Input: part model. Units: mm. Frame: model coordinates. A direction names the side the tool comes from. Coordinates: 2 decimals unless noted, no trailing zeros. Order: outer loops, then holes, each group sorted by start corner. A loop starts at its lowest first (then second) coordinate and runs counter-clockwise, first axis right, second up. Notation, with made-up numbers: M 60,23 L 87,23 A33 ccw 87,56 Z; hole C -39.75,18 d5. An arc over 180 degrees is marked long. One line per item, written item: value.
```python
from build123d import *

# Parameters (mm, degrees)
F0_W        = 16
F0_H        = 22
F0_W_2      = 4
F0_H_2      = 9
F1_DEPTH    = 3
F2_DEPTH    = 15
F3_DEPTH    = 2.5
F4_DEPTH    = 2.5
F5_T1_DEPTH = 3
F5_T3_DEPTH = 25
F7_W        = 4
F7_H        = 9
F8_DEPTH    = 1
F10_DEPTH   = 1
F11_R       = 5


# Not quite as in the source:
# - a fillet or chamfer that OpenCascade refuses, or shapes differently, is made with other operations: its cross-section is extruded or revolved along the edge and cut away or added
# - two fillets or chamfers of one size are made in one step


with BuildPart() as f1:
    # F0 (on Top) → F1 (new body)
    with BuildSketch(Plane.XY):
        with Locations((8, 11)):
            Rectangle(F0_W, F0_H)
        with Locations((6, 9.5)):
            Rectangle(F0_W_2, F0_H_2, mode=Mode.SUBTRACT)
        with Locations((24, 11)):
            Rectangle(F0_W, F0_H)
        with Locations((26, 9.5)):
            Rectangle(F0_W_2, F0_H_2, mode=Mode.SUBTRACT)
    extrude(amount=F1_DEPTH)

    # F0 (on Top) → F2 (join)
    with BuildSketch(Plane.XY):
        Polygon((0, 27), (0, 23), (3, 23), (3, 25.5), (8, 25.5), (8, 27), align=None)
        Polygon((0, 23), (0, 22), (16, 22), (16, 23), (3, 23), align=None)
        Polygon((16, 23), (16, 22), (32, 22), (32, 23), (29, 23), align=None)
        Polygon((29, 23), (32, 23), (32, 27), (24, 27), (24, 25.5), (29, 25.5), align=None)
    extrude(amount=F2_DEPTH)

    # F3 (add): a face of the model
    f3_faces = [f1.faces().sort_by_distance(p)[0] for p in [
        (32, 0.3088689042, 1.5),
    ]]
    extrude(f3_faces, amount=F3_DEPTH)

    # F4 (add): a face of the model
    f4_faces = [f1.faces().sort_by_distance(p)[0] for p in [
        (0, 0.3088689042, 1.5),
    ]]
    extrude(f4_faces, amount=F4_DEPTH)

    # F5: fillet of radius 2 on 10 edges, made by hand

    # F5_s2 → F5_t1 (join)
    with BuildSketch(Plane.XY):
        with BuildLine():
            ThreePointArc((28, 12), (27.4142135624, 13.4142135624), (26, 14))
            Line((26, 14), (28, 14))
            Line((28, 14), (28, 12))
        make_face()
        with BuildLine():
            ThreePointArc((28, 7), (27.4142135624, 5.5857864376), (26, 5))
            Line((26, 5), (28, 5))
            Line((28, 5), (28, 7))
        make_face()
        with BuildLine():
            ThreePointArc((26, 14), (24.5857864376, 13.4142135624), (24, 12))
            Line((24, 12), (24, 14))
            Line((24, 14), (26, 14))
        make_face()
        with BuildLine():
            ThreePointArc((24, 7), (24.5857864376, 5.5857864376), (26, 5))
            Line((26, 5), (24, 5))
            Line((24, 5), (24, 7))
        make_face()
        with BuildLine():
            ThreePointArc((8, 12), (7.4142135624, 13.4142135624), (6, 14))
            Line((6, 14), (8, 14))
            Line((8, 14), (8, 12))
        make_face()
        with BuildLine():
            ThreePointArc((8, 7), (7.4142135624, 5.5857864376), (6, 5))
            Line((6, 5), (8, 5))
            Line((8, 5), (8, 7))
        make_face()
        with BuildLine():
            ThreePointArc((6, 14), (4.5857864376, 13.4142135624), (4, 12))
            Line((4, 12), (4, 14))
            Line((4, 14), (6, 14))
        make_face()
        with BuildLine():
            ThreePointArc((4, 7), (4.5857864376, 5.5857864376), (6, 5))
            Line((6, 5), (4, 5))
            Line((4, 5), (4, 7))
        make_face()
    extrude(amount=F5_T1_DEPTH)

    # F5_s4 → F5_t3 (cut)
    with BuildSketch(Plane.XY.offset(-5)):
        with BuildLine():
            ThreePointArc((32.5, 27), (33.9142135624, 26.4142135624), (34.5, 25))
            Line((34.5, 25), (34.5, 27))
            Line((34.5, 27), (32.5, 27))
        make_face()
        with BuildLine():
            ThreePointArc((-0.5, 27), (-1.9142135624, 26.4142135624), (-2.5, 25))
            Line((-2.5, 25), (-2.5, 27))
            Line((-2.5, 27), (-0.5, 27))
        make_face()
    extrude(amount=F5_T3_DEPTH, mode=Mode.SUBTRACT)

    # F7 (on face) → F8 (cut)
    with BuildSketch(Plane.XY):
        with BuildLine():
            Line((2.7, 12), (2.7, 7))
            ThreePointArc((2.7000000011, 7), (6, 3.7000000011), (9.2999999989, 7))
            Line((9.3, 7), (9.3, 12))
            ThreePointArc((9.3, 12), (6, 15.3), (2.7, 12))
        make_face()
        with Locations((6, 9.5)):
            Rectangle(F7_W, F7_H, mode=Mode.SUBTRACT)
        with Locations((6, 9.5)):
            Rectangle(F7_W, F7_H)
    extrude(amount=F8_DEPTH, mode=Mode.SUBTRACT)

    # F9 (on face) → F10 (cut)
    with BuildSketch(Plane.XY):
        with BuildLine():
            Line((22.7, 12), (22.7, 7))
            ThreePointArc((22.7, 7), (26, 3.7), (29.3, 7))
            Line((29.3, 7), (29.3, 12))
            ThreePointArc((29.3, 12), (26, 15.3), (22.7, 12))
        make_face()
    extrude(amount=F10_DEPTH, mode=Mode.SUBTRACT)

    # F11
    f11_edges = [f1.edges().sort_by_distance(p)[0] for p in [
        (34.5, 0, 1.5),
        (-2.5, 0, 1.5),
    ]]
    fillet(f11_edges, radius=F11_R)


solid = f1.part
```
(1) Cut plane B-B on z = 11.25. Output: boundary loops of the cut face in (x, y).
Data:
outline: M -2.5,22 L 34.5,22 L 34.5,25 A2 ccw 32.5,27 L 24,27 L 24,25.5 L 29,25.5 L 29,23 L 3,23 L 3,25.5 L 8,25.5 L 8,27 L -0.5,27 A2 ccw -2.5,25 Z
(2) Cut plane A-A on x = 7.5. Output: boundary loops of the cut face in (y, z).
Data:
outline: M 0,0 L 4.06,0 L 4.06,1 L 5.68,1 L 5.68,3 L 0,3 Z; M 13.32,1 L 14.94,1 L 14.94,0 L 23,0 L 23,15 L 22,15 L 22,3 L 13.32,3 Z; M 25.5,0 L 27,0 L 27,15 L 25.5,15 Z
(3) Draft query along Y for faces 5 (the flat face through (34.5, 18, 1)), 6 (the cylindrical face through (33.07, 1.5, 1.52)), 7 (the flat face through (26, 25.5, 7)). Return one class per face: released by +Y, released by -Y, zero draft, split by the parting line, or undercut.
Data:
face 5: zero draft
face 6: released by -Y
face 7: undercut
(4) Cut plane C-C on x = 11.5. Output: boundary loops of the cut face in (y, z), plus the area to 3 significant figures.
Data:
outline: M 0,0 L 23,0 L 23,15 L 22,15 L 22,3 L 0,3 Z
area: 81.0 mm2
(5) Ray query, line 1 (X direction, y = 8.75, z = 1.75); line 2 (X direction, y = 24.5, z = 2.5); line 3 (Y direction, x = 28.5, z = 11.5). Return the intervals inside material, ascending. Write a range as from..to.
Data:
line 1: x = -2.5..4, 8..24, 28..34.5
line 2: x = -2.5..3, 29..34.5
line 3: y = 22..23, 25.5..27
(6) First-contact query: pin 1 (0.8 mm diameter, centred on y = 26.5, z = 11, fed in from +X); pin 2 (2 mm diameter, centred on x = 19, y = 15, fed in from +Z); pin 3 (2.5 mm diameter, centred on x = 6.5, z = 9.5, fed in from -Y). Flat tips, straight axial feed; report the tip coordinate or a pass-through.
Data:
pin 1: stops at x = 34.17
pin 2: stops at z = 3
pin 3: stops at y = 22
(7) Cut plane D-D on y = 19.75. Output: boundary loops of the cut face in (x, z), plus the area to 3 significant figures.
Data:
outline: M -2.5,0 L 34.5,0 L 34.5,3 L -2.5,3 Z
area: 111 mm2
(8) Access query for faces 1 (the flat face through (8, 26, 7)), 2 (the cylindrical face through (25.9, 3.7, 0.5)), 3 (the flat face through (16, 23, 7)), 4 (the flat face through (28, 27, 7)). Directions: +Z, -Z, +X, -X, +Y, -Y. A direction counts if a zero-diameter tool reaches every point of the face in a straight line with its end or side. Return the directions, or none.
Data:
face 1: +Z, -Z, +Y
face 2: -Z
face 3: +Z, -Z
face 4: +Z, -Z, +X, -X, +Y
